from build123d import *

# Parameters (mm, degrees)
F0_W        = 95
F0_H        = 32
F1_DEPTH    = 20
F3_R        = 5
F4_R        = 5
F6_DEPTH    = 25
F7_DEPTH    = 47.1
F8_T        = 2.5
F8_T3_DEPTH = 23.9149246247
F8_T5_DEPTH = 23.2696171533
F8_T8_ANGLE = 58.1590270575
F9_W        = 21
F9_H        = 10
F10_DEPTH   = 16.1
F13_DEPTH   = 25


# Not quite as in the source:
# - a shell that OpenCascade refuses in one call is made with other operations: the cavity is built on its own and cut out


with BuildPart() as f1:
    # F0 (on Top) → F1 (new body)
    with BuildSketch(Plane.XY):
        with Locations((66.9030988216, -21.9037037492)):
            Rectangle(F0_W, F0_H)
    extrude(amount=F1_DEPTH)

    # F3
    f3_edges = [f1.edges().sort_by_distance(p)[0] for p in [
        (66.903099, -37.903704, 20),
    ]]
    fillet(f3_edges, radius=F3_R)

    # F4
    f4_edges = [f1.edges().sort_by_distance(p)[0] for p in [
        (66.903099, -5.903704, 20),
    ]]
    fillet(f4_edges, radius=F4_R)

    # F5 (on face) → F6 (cut)
    with BuildSketch(Plane.XY.offset(20)):
        Polygon((101.4030988216, -20.6582732499), (101.4030988216, -10.9037037492), (80.4030988216, -10.9037037492), (80.4030988216, -20.9037037492), (101.4030988216, -20.9037037492), align=None)
    extrude(amount=-F6_DEPTH, mode=Mode.SUBTRACT)

    # F2 (on face) → F7 (cut)
    with BuildSketch(Plane.YZ.offset(114.4030988216)):
        with BuildLine():
            ThreePointArc((-37.9037037492, 12.3313413933), (-22.4823614594, 18.7362249856), (-5.9037037492, 16.7391169816))
            Line((-5.9037037492, 16.7391169816), (-5.9037037492, 20))
            Line((-5.9037037492, 20), (-37.9037037492, 20))
            Line((-37.9037037492, 20), (-37.9037037492, 12.3313413933))
        make_face()
    extrude(amount=-F7_DEPTH, mode=Mode.SUBTRACT)

    # F8: shell of thickness 2.5, made by hand


with BuildPart() as f8_core1:
    # F8_t2: copy of F1
    add(f1.part)

    # the walls: a layer under each face that stays
    f8_faces = [f8_core1.faces().sort_by_distance(p)[0] for p in [
        (19.4030988216, -21.9037037492, 10),
        (43.3530988216, -21.9037037492, 20),
        (66.9030988216, -7.3681698432, 18.5355339059),
        (43.3530988216, -36.4392376551, 18.5355339059),
        (66.9030988216, -5.9037037492, 7.5),
        (66.9030988216, -37.9037037492, 7.5),
        (67.3030988216, -32.6316572711, 16.1656706966),
        (90.8530988216, -22.6776915616, 18.7087222914),
        (114.4030988216, -21.9037037492, 9.5218727657),
        (80.4030988216, -15.9037037492, 9.5218727657),
        (90.9030988216, -20.9037037492, 9.4574623123),
        (101.4030988216, -15.9037037492, 9.5218727657),
        (90.9030988216, -10.9037037492, 9.1348085767),
    ]]
    thicken(f8_faces, amount=-F8_T, mode=Mode.SUBTRACT)

    # F8_s4 → F8_t3 (cut)
    with BuildSketch(Plane.XY.offset(-2.5)):
        Polygon((80.4280988216, -20.8787037492), (77.9030988216, -20.9037037492), (77.9030988216, -23.4037037492), (80.4030988216, -23.4037037492), align=None)
        Polygon((101.3780988216, -20.8787037492), (101.4030988216, -23.4037037492), (103.9030988216, -23.4037037492), (103.9030988216, -20.9037037492), align=None)
    extrude(amount=F8_T3_DEPTH, mode=Mode.SUBTRACT)

    # F8_s6 → F8_t5 (cut)
    with BuildSketch(Plane.XY.offset(-2.5)):
        Polygon((80.4280988216, -10.9287037492), (77.9030988216, -10.9037037492), (77.9030988216, -8.4037037492), (80.4030988216, -8.4037037492), align=None)
        Polygon((101.3780988216, -10.9287037492), (103.9030988216, -10.9037037492), (103.9030988216, -8.4037037492), (101.4030988216, -8.4037037492), align=None)
    extrude(amount=F8_T5_DEPTH, mode=Mode.SUBTRACT)

    # F8_s7 → F8_t8 (revolve, cut)
    with BuildSketch(Plane(origin=(0, -18.0639523955, -13.7441213447), x_dir=(1, 0, 0), z_dir=(0, -0.7958327334, -0.6055165237))):
        Polygon((67.3280988216, 32.7900040558), (64.8030988216, 32.7650040558), (64.8030988216, 30.2650040558), (67.3030988216, 30.2650040558), align=None)
    revolve(axis=Axis((67.3030988216, -17.9961461515, -13.8332393562), (-1, 0, 0)), revolution_arc=F8_T8_ANGLE, mode=Mode.SUBTRACT)


with BuildPart() as f1_1:
    add(f1.part)

    # what is left inside the walls is the cavity
    f8_cavity = [f8_core1.part.solids().sort_by_distance(p)[0] for p in [
        (66.903099, -26.403704, 0.025),
    ]]
    add(f8_cavity, mode=Mode.SUBTRACT)

    # F9 (on face) → F10 (cut)
    with BuildSketch(Plane(origin=(0, 0, 0), x_dir=(1, 0, 0), z_dir=(0, 0, -1))):
        Polygon((77.9030988216, 10.9037037492), (77.9030988216, 8.4037037492), (103.9030988216, 8.4037037492), (103.9030988216, 10.9037037492), (103.9030988216, 20.9037037492), (103.9030988216, 23.4037037492), (77.9030988216, 23.4037037492), (77.9030988216, 20.9037037492), align=None)
        with Locations((90.9030988216, 15.9037037492)):
            Rectangle(F9_W, F9_H, mode=Mode.SUBTRACT)
    extrude(amount=-F10_DEPTH, mode=Mode.SUBTRACT)

    # F12 (on face) → F13 (cut)
    with BuildSketch(Plane.XZ.offset(37.9037037492)):
        Polygon((46.4005000293, 6), (32.4030988216, 6), (32.4030988216, 2.1138605662), (32.4005000293, 2.1138605662), (32.4005000293, 0), (46.4005000293, 0), align=None)
    extrude(amount=-F13_DEPTH, mode=Mode.SUBTRACT)


solid = f1_1.part
The listing builds one solid part. Answer for the finished solid, in the listing's coordinates (mm). A direction names the side the tool comes from. Round coordinates to 2 decimals unless told otherwise and drop trailing zeros. Write each loop counter-clockwise with the first axis right and the second up, starting at its lowest first coordinate (ties: lowest second). Pieces come first, ordered by that corner, then holes. Notation, with made-up numbers: (73.25, 13) - (104.25, 13) arc R16 ccw to (104.25, 42) - close; hole circle Ø11 at (80.25, -6.75). An arc over 180 degrees is marked (long way). Use a Markdown table: item, result. Add a question column.
1. A tool of negligible diameter and unlimited length cuts with its end or side. For faces 1 (the face through (91, -20.904, 18)), 2 (the face through (32.403, -37, 4)), 3 (the face through (91, -23, 16.1)), 4 (the face through (91.183, -22.909, 18.675)), 5 (the face through (19.403, -22, 10)), from which of +Z, -Z, +X, -X, +Y, -Y can it reach the whole face along a straight path? Write none if from no direction.
2. The part is cut by section D-D (y = -17.5). Write down the section's boundary in (x, z).
3. Consider line 1 (X direction, y = -19, z = 7); line 2 (Y direction, x = 75, z = 2.5); line 3 (X direction, y = -25, z = 17). Determine where each line is inside the solid, lowest interval first.
4. The part is cut by section C-C (x = 63.5). Write down the section's boundary in (y, z), and give its area (3 significant figures).
5. The part is cut by section A-A (x = 98). Write down the section's boundary in (y, z), and give its area (3 significant figures).
6. The part is cut by section B-B (z = 3.5). Write down the section's boundary in (x, y), and give its area (3 significant figures).
7. Flat-ended cylindrical pins translate along their axes: P1, Ø0.7, axis at x = 38.5, y = -37, coming from the -Z side; P2, Ø4, axis at x = 99.5, y = -33.5, coming from the +Z side; P3, Ø10, axis at x = 56, y = -16, coming from the -Z side. Find the tip coordinate at first contact, or state that the pin passes through.
Reported:
| question | item | result |
|---|---|---|
| 1 | face 1 | +Z, -Z |
| 1 | face 2 | -Z, -Y |
| 1 | face 3 | -Z |
| 1 | face 4 | +Z, +X |
| 1 | face 5 | +Z, -Z, -X, +Y, -Y |
| 2 | outline | (19.4, 0) - (21.9, 0) - (21.9, 17.5) - (64.8, 17.5) - (64.8, 16.54) - (77.9, 16.54) - (77.9, 16.1) - (80.4, 16.1) - (80.4, 19.04) - (67.3, 19.04) - (67.3, 20) - (19.4, 20) - close; (101.4, 16.1) - (103.9, 16.1) - (103.9, 16.54) - (111.9, 16.54) - (111.9, 0) - (114.4, 0) - (114.4, 19.04) - (101.4, 19.04) - close |
| 3 | line 1 | 19.4 to 21.9, 111.9 to 114.4 |
| 3 | line 2 | -37.9 to -35.4, -8.4 to -5.9 |
| 3 | line 3 | 19.4 to 21.9, 64.8 to 114.4 |
| 4 | outline | (-37.9, 0) - (-35.4, 0) - (-35.4, 15) arc R2.5 cw to (-32.9, 17.5) - (-10.9, 17.5) arc R2.5 cw to (-8.4, 15) - (-8.4, 0) - (-5.9, 0) - (-5.9, 15) arc R5 ccw to (-10.9, 20) - (-32.9, 20) arc R5 ccw to (-37.9, 15) - close |
| 4 | area | 159 mm^2 |
| 5 | outline | (-37.9, 0) - (-35.4, 0) - (-35.4, 11.06) arc R30.38 cw to (-23.4, 16.06) - (-23.4, 16.1) - (-20.9, 16.1) - (-20.9, 18.91) arc R32.88 ccw to (-37.9, 12.33) - close; (-10.9, 16.1) - (-8.4, 16.1) - (-8.4, 0) - (-5.9, 0) - (-5.9, 15) arc R5 ccw to (-6.27, 16.88) arc R32.88 ccw to (-10.9, 18.27) - close |
| 5 | area | 120 mm^2 |
| 6 | outline | (19.4, -37.9) - (32.4, -37.9) - (32.4, -35.4) - (21.9, -35.4) - (21.9, -8.4) - (111.9, -8.4) - (111.9, -35.4) - (46.4, -35.4) - (46.4, -37.9) - (114.4, -37.9) - (114.4, -5.9) - (19.4, -5.9) - close |
| 6 | area | 575 mm^2 |
| 7 | P1 | z = 6 |
| 7 | P2 | z = 16.14 |
| 7 | P3 | z = 17.5 |
